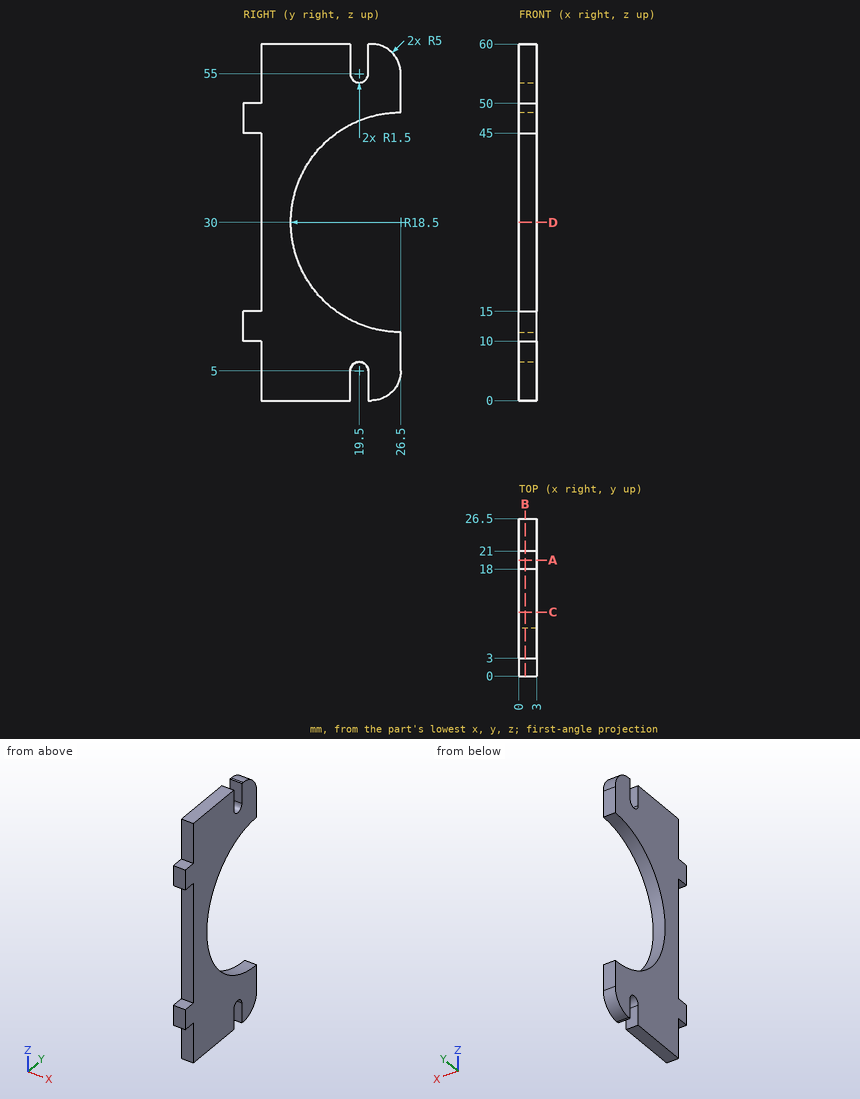
The drawing under review shows one solid part. Ordinate dimensions are in mm from its lowest x, y, z. Give positions to 0.01 mm unless a question says otherwise; leave off trailing zeros. Write each loop counter-clockwise with the first axis right and the second up, starting at its lowest first coordinate (ties: lowest second). Pieces come first, ordered by that corner, then holes. Notation, with made-up numbers: (50, 7) -> (68, 7) arc R22 cw to (68, 34) -> close; hole circle Ø5 at (19, 56.25). An arc over 180 degrees is marked (long way). Answer in a Markdown table with one row per item.
(1) Clearance check with flat-ended pins moving along their axes: pin 1 (0.9 mm diameter, centred on x = 1.5, y = 1, fed in from +Z); pin 2 (0.9 mm diameter, centred on x = 2, z = 2.5, fed in from +Y); pin 3 (1 mm diameter, centred on x = 2, z = 29.5, fed in from -Y). State where each tip first meets the part, or that it passes through.
Results:
| item | result |
|---|---|
| pin 1 | z = 50 |
| pin 2 | y = 26.06 |
| pin 3 | y = 3 |
(2) Consider section C-C (y = 10.75). State the section outline as (x, z) points.
Results:
| item | result |
|---|---|
| outline | (0, 0) -> (3, 0) -> (3, 20.29) -> (0, 20.29) -> close; (0, 39.71) -> (3, 39.71) -> (3, 60) -> (0, 60) -> close |
(3) Consider section A-A (y = 19.5). State the section outline as (x, z) points.
Results:
| item | result |
|---|---|
| outline | (0, 6.5) -> (3, 6.5) -> (3, 12.88) -> (0, 12.88) -> close; (0, 47.12) -> (3, 47.12) -> (3, 53.5) -> (0, 53.5) -> close |
(4) Consider section D-D (z = 30). State the section outline as (x, y) points, then the cut area to 3 significant figures.
Results:
| item | result |
|---|---|
| outline | (0, 3) -> (3, 3) -> (3, 8) -> (0, 8) -> close |
| area | 15.0 mm2 |
(5) Consider section B-B (x = 1.05). State the section outline as (y, z) points.
Results:
| item | result |
|---|---|
| outline | (0, 10) -> (3, 10) -> (3, 0) -> (18, 0) -> (18, 5) arc R1.5 cw to (21, 5) -> (21, 0) -> (21.5, 0) arc R5 ccw to (26.5, 5) -> (26.5, 11.5) arc R18.5 cw to (26.5, 48.5) -> (26.5, 55) arc R5 ccw to (21.5, 60) -> (21, 60) -> (21, 55) arc R1.5 cw to (18, 55) -> (18, 60) -> (3, 60) -> (3, 50) -> (0, 50) -> (0, 45) -> (3, 45) -> (3, 15) -> (0, 15) -> close |
(6) To check wall thickness, follow probe 1 along Y at (x, z) = (2.45, 7.5); probe 2 along Z at (x, y) = (1.55, 23.75); probe 3 along Z at (x, y) = (1.75, 25). State the ranges of each line that lie inside material, in increasing order.
Results:
| item | result |
|---|---|
| probe 1 | 3 to 26.5 |
| probe 2 | 0.53 to 11.71, 48.29 to 59.47 |
| probe 3 | 1.43 to 11.56, 48.44 to 58.57 |
